Here's the drawing with two shaded views (mm, measured from the low corner). I have some questions. A direction names the side the tool comes from. Round coordinates to 2 decimals unless told otherwise and drop trailing zeros. Loops run counter-clockwise (first coordinate to the right, second up) from the corner with the lowest first, then second, coordinate; pieces in that order, holes last. Notation, with made-up numbers: M 61,68.25 L 70,68.25 A29 cw 70,103.25 Z; hole C 68,82 d2. An arc over 180 degrees is marked long. One line per item, written item: value. Start each with the question number.
Q1. Imagine slicing it at B-B (y = 63.5). Please give me the cut outline in (x, z).
Q2. I'm going to push flat-ended pins straight in: pin 1 Ø11.5 at (x, z) = (17.5, 19) entering from +Y; pin 2 Ø8 at (x, z) = (17.5, 13) entering from -Y; pin 3 Ø6 at (y, z) = (63.5, 30.5) entering from +X. Where does each tip first touch, or does it pass through?
Q3. Please list where these lines run through material, in increasing order: line 1 along X through (y, z) = (2.3, 21); line 2 along Y through (x, z) = (1.3, 5.5); line 3 along Z through (x, y) = (25, 2.1).
Q4. Imagine slicing it at D-D (x = 12). Please give me the cut outline in (y, z), then the cut area to 3 significant figures.
Q5. Which directions (+Z, -Z, +X, -X, +Y, -Y) give clear straight access to the entire face, cutting with the end or side of a thin tool? Please do the marked faces 1 and 2.
Q6. Imagine slicing it at C-C (z = 21). Please give me the cut outline in (x, y).
Q7. Imagine slicing it at A-A (x = 25). Please give me the cut outline in (y, z).
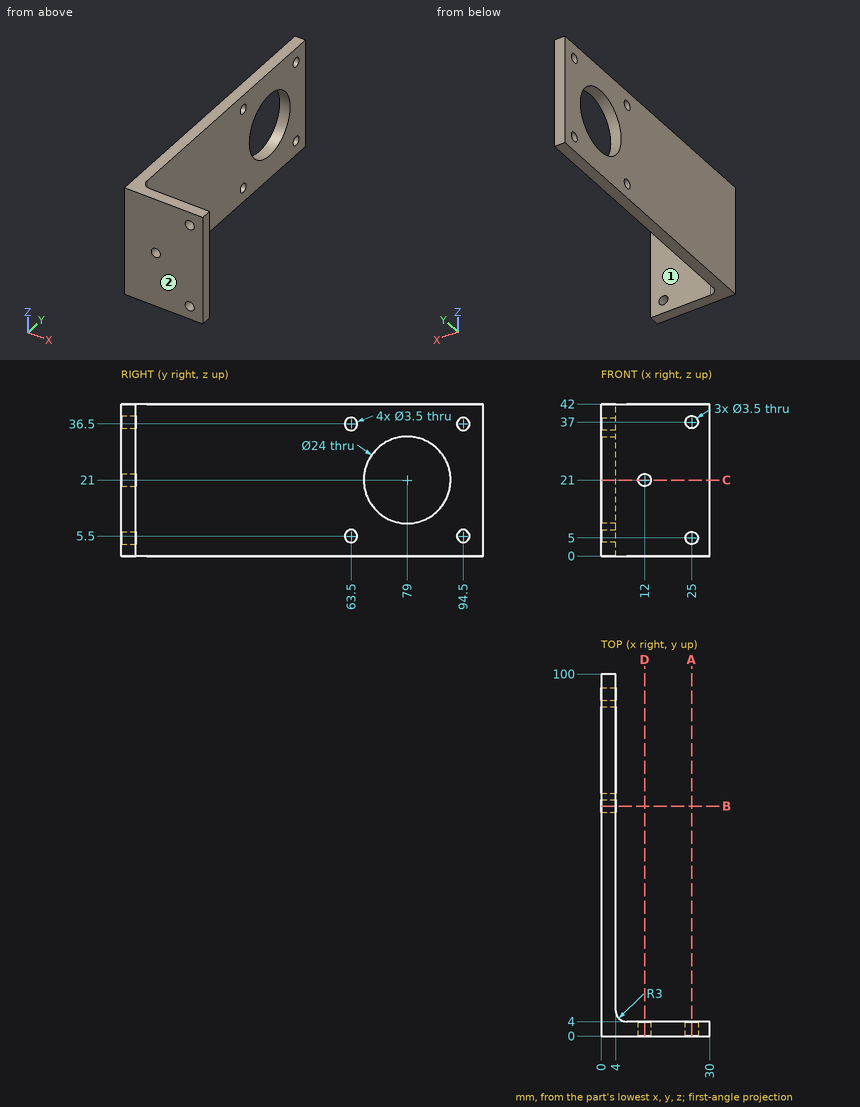
Report:
1. outline: M 0,0 L 4,0 L 4,3.75 L 0,3.75 Z; M 0,7.25 L 4,7.25 L 4,34.75 L 0,34.75 Z; M 0,38.25 L 4,38.25 L 4,42 L 0,42 Z
2. pin 1: stops at y = 4
2. pin 2: stops at y = 0
2. pin 3: stops at x = 4
3. line 1: x = 0 to 10.25, 13.75 to 30
3. line 2: y = 0 to 61.75, 65.25 to 92.75, 96.25 to 100
3. line 3: z = 0 to 3.25, 6.75 to 35.25, 38.75 to 42
4. outline: M 0,0 L 4,0 L 4,19.25 L 0,19.25 Z; M 0,22.75 L 4,22.75 L 4,42 L 0,42 Z
4. area: 154 mm²
5. face 1: +Z, -Z, +X, +Y
5. face 2: +Z, -Z, +X, -X, -Y
6. outline: M 0,0 L 10.25,0 L 10.25,4 L 7,4 A3 cw 4,7 L 4,67 L 0,67 Z; M 0,91 L 4,91 L 4,100 L 0,100 Z; M 13.75,0 L 30,0 L 30,4 L 13.75,4 Z
7. outline: M 0,0 L 4,0 L 4,3.25 L 0,3.25 Z; M 0,6.75 L 4,6.75 L 4,35.25 L 0,35.25 Z; M 0,38.75 L 4,38.75 L 4,42 L 0,42 Z
